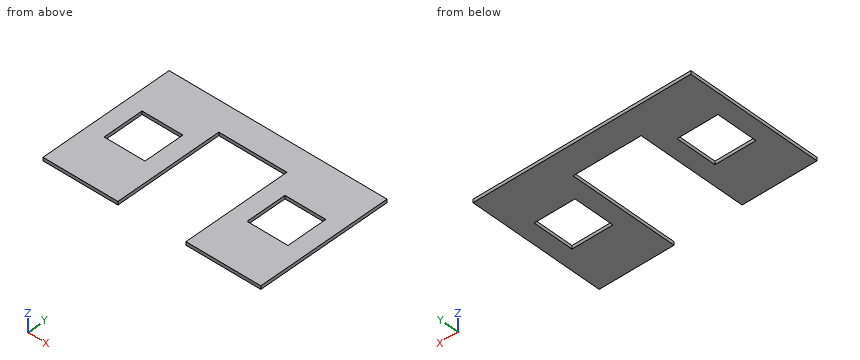
```python
from build123d import *

# Parameters (mm, degrees)
SKETCH1_W           = 406.4
SKETCH1_H           = 254
BOSS_EXTRUDE1_DEPTH = 6.35
CUT_EXTRUDE1_REACH  = 8.35
SKETCH2_W           = 127
SKETCH2_H           = 203.2
CUT_EXTRUDE3_REACH  = 8.35
SKETCH3_W           = 76.2
SKETCH3_H           = 76.2
CUT_EXTRUDE4_REACH  = 8.35
SKETCH4_W           = 76.2
SKETCH4_H           = 76.2


with BuildPart() as part:
    # Sketch1 → Boss-Extrude1 (new body)
    with BuildSketch(Plane.XY):
        with Locations((0, 127)):
            Rectangle(SKETCH1_W, SKETCH1_H)
    extrude(amount=BOSS_EXTRUDE1_DEPTH)

    # Sketch2 → Cut-Extrude1 (cut, up to next)
    with BuildSketch(Plane.XY.offset(6.35), mode=Mode.PRIVATE) as cut_extrude1_sk1:
        with Locations((0, 101.6)):
            Rectangle(SKETCH2_W, SKETCH2_H)
    cut_extrude1_tool1 = extrude(cut_extrude1_sk1.sketch, amount=-CUT_EXTRUDE1_REACH, mode=Mode.PRIVATE) & part.part
    add(cut_extrude1_tool1.solids().sort_by_distance((0, 101.6, 6.35))[0], mode=Mode.SUBTRACT)

    # Sketch3 → Cut-Extrude3 (cut, up to next)
    with BuildSketch(Plane.XY.offset(6.35), mode=Mode.PRIVATE) as cut_extrude3_sk1:
        with Locations((-133.35, 127)):
            Rectangle(SKETCH3_W, SKETCH3_H)
    cut_extrude3_tool1 = extrude(cut_extrude3_sk1.sketch, amount=-CUT_EXTRUDE3_REACH, mode=Mode.PRIVATE) & part.part
    add(cut_extrude3_tool1.solids().sort_by_distance((-133.35, 127, 6.35))[0], mode=Mode.SUBTRACT)

    # Sketch4 → Cut-Extrude4 (cut, up to next)
    with BuildSketch(Plane.XY.offset(6.35), mode=Mode.PRIVATE) as cut_extrude4_sk1:
        with Locations((133.35, 127)):
            Rectangle(SKETCH4_W, SKETCH4_H)
    cut_extrude4_tool1 = extrude(cut_extrude4_sk1.sketch, amount=-CUT_EXTRUDE4_REACH, mode=Mode.PRIVATE) & part.part
    add(cut_extrude4_tool1.solids().sort_by_distance((133.35, 127, 6.35))[0], mode=Mode.SUBTRACT)


solid = part.part
```
For this review, take the finished solid that the model builds, in its own axes (mm). Coordinates: 2 decimals unless noted, no trailing zeros. Order: outer loops, then holes, each group sorted by start corner. A loop starts at its lowest first (then second) coordinate and runs counter-clockwise, first axis right, second up. Notation, with made-up numbers: (-15.75, -36) -> (34.25, -36) arc R24 ccw to (34.25, -10) -> close; hole circle Ø10 at (68, -30.75). An arc over 180 degrees is marked (long way). Use CSV: the item, a comma, the result in double quotes. Start each with the question number.
Item 1: We need section B-B, the plane y = 28. Give the boundary of the cut face in (x, z), then the cut area to 3 significant figures.
Item 2: We need section A-A, the plane x = -142.5. Give the boundary of the cut face in (y, z).
Item 3: We need section C-C, the plane y = 136. Give the boundary of the cut face in (x, z).
Item 4: We need section D-D, the plane z = 5. Give the boundary of the cut face in (x, y), then the cut area to 3 significant figures.
Item 5: Wall thickness on probe 1 along X at (y, z) = (142.5, 1); probe 2 along X at (y, z) = (14, 4.5); probe 3 along Y at (x, z) = (-123, 1): over which ranges is each line inside the solid? List them lowest first.
Item 6: Insertion check: pin 1 (3 mm diameter, centred on x = 137, z = 3.5, fed in from -Y); pin 2 (3 mm diameter, centred on x = -30, z = 2.5, fed in from -Y). Each pin has a flat end and moves straight along its axis. Give the tip position at first contact, or say it passes through.
Derived:
1,outline,"(-203.2, 0) -> (-63.5, 0) -> (-63.5, 6.35) -> (-203.2, 6.35) -> close; (63.5, 0) -> (203.2, 0) -> (203.2, 6.35) -> (63.5, 6.35) -> close"
1,area,"1,770 mm^2"
2,outline,"(0, 0) -> (88.9, 0) -> (88.9, 6.35) -> (0, 6.35) -> close; (165.1, 0) -> (254, 0) -> (254, 6.35) -> (165.1, 6.35) -> close"
3,outline,"(-203.2, 0) -> (-171.45, 0) -> (-171.45, 6.35) -> (-203.2, 6.35) -> close; (-95.25, 0) -> (-63.5, 0) -> (-63.5, 6.35) -> (-95.25, 6.35) -> close; (63.5, 0) -> (95.25, 0) -> (95.25, 6.35) -> (63.5, 6.35) -> close; (171.45, 0) -> (203.2, 0) -> (203.2, 6.35) -> (171.45, 6.35) -> close"
4,outline,"(-203.2, 0) -> (-63.5, 0) -> (-63.5, 203.2) -> (63.5, 203.2) -> (63.5, 0) -> (203.2, 0) -> (203.2, 254) -> (-203.2, 254) -> close; hole (-171.45, 88.9) -> (-95.25, 88.9) -> (-95.25, 165.1) -> (-171.45, 165.1) -> close; hole (95.25, 88.9) -> (171.45, 88.9) -> (171.45, 165.1) -> (95.25, 165.1) -> close"
4,area,"65,800 mm^2"
5,probe 1,"x = -203.2 to -171.45, -95.25 to -63.5, 63.5 to 95.25, 171.45 to 203.2"
5,probe 2,"x = -203.2 to -63.5, 63.5 to 203.2"
5,probe 3,"y = 0 to 88.9, 165.1 to 254"
6,pin 1,"stops at y = 0"
6,pin 2,"stops at y = 203.2"
